from build123d import *

# Parameters (mm, degrees)
EXTRUDE_1_DEPTH = 10
SKETCH_2_R      = 10
EXTRUDE_2_DEPTH = 10


with BuildPart() as part:
    # 스케치1 → 보스-돌출1 (new body)
    with BuildSketch(Plane.XY):
        with BuildLine():
            Line((0, 20), (-82.363877474, 20))
            Line((-82.363877474, 20), (-82.363877474, -20))
            Line((-82.363877474, -20), (0, -20))
            ThreePointArc((0, -20), (20, 0), (0, 20))
        make_face()
    extrude(amount=EXTRUDE_1_DEPTH)

    # 스케치2 → 보스-돌출2 (add)
    with BuildSketch(Plane.XY.offset(10)):
        with Locations((0, -0.593223752)):
            Circle(SKETCH_2_R)
    extrude(amount=EXTRUDE_2_DEPTH)


solid = part.part
Build history of the part. All positions in model axes, mm. A direction names the side the tool comes from. Round coordinates to 2 decimals unless told otherwise and drop trailing zeros. Loops run counter-clockwise (first coordinate to the right, second up) from the corner with the lowest first, then second, coordinate; pieces in that order, holes last. Notation, with made-up numbers: (83.25, 29.25) -> (128.25, 29.25) arc R25 ccw to (128.25, 44.25) -> close; hole circle Ø2 at (-35.5, 55). An arc over 180 degrees is marked (long way). Use CSV: the item, a comma, the result in double quotes. Start each with the question number.
Q1. Saw through at A-A on x = 3.5. Give the cut face in (y, z), and give its area (3 significant figures).
Q2. Drill centre lines: L1, parallel to Z at x = -29.5, y = 13.5; L2, parallel to X at y = -0.5, z = 16; L3, parallel to X at y = 7, z = 7.5 (3 decimals). Where is each one in solid material? Low to high.
Q3. Saw through at D-D on x = -68.5. Give the cut face in (y, z).
Q4. Which spindle directions (+Z, -Z, +X, -X, +Y, -Y) get a long thin tool onto all of the face, cutting with end or side? Do faces 1 (the face through (-42, -20, 5)), 2 (the face through (-2.168, -10.355, 14.93)). Say none if no direction does.
Q5. Flat gauge pins, fed straight in: pin 1 Ø10 at (x, y) = (-53, 3.5) entering from +Z; pin 2 Ø1.5 at (y, z) = (10.5, 4) entering from +X; pin 3 Ø12 at (x, z) = (-15.5, 14.5) entering from +Y. Where does each tip first touch, or does it go through?
Q6. Saw through at C-C on z = 9. Give the cut face in (x, y), and give its area (3 significant figures).
Q7. Saw through at B-B on y = -2. Give the cut face in (x, z).
Solutions:
1,outline,"(-19.69, 0) -> (19.69, 0) -> (19.69, 10) -> (8.77, 10) -> (8.77, 20) -> (-9.96, 20) -> (-9.96, 10) -> (-19.69, 10) -> close"
1,area,"581 mm^2"
2,L1,"z = 0 to 10"
2,L2,"x = -10 to 10"
2,L3,"x = -82.364 to 18.735"
3,outline,"(-20, 0) -> (20, 0) -> (20, 10) -> (-20, 10) -> close"
4,face 1,"+Z, -Z, +X, -X, -Y"
4,face 2,"+Z"
5,pin 1,"stops at z = 10"
5,pin 2,"stops at x = 17.46"
5,pin 3,"stops at y = 20"
6,outline,"(-82.36, -20) -> (0, -20) arc R20 ccw to (0, 20) -> (-82.36, 20) -> close"
6,area,"3,920 mm^2"
7,outline,"(-82.36, 0) -> (19.9, 0) -> (19.9, 10) -> (9.9, 10) -> (9.9, 20) -> (-9.9, 20) -> (-9.9, 10) -> (-82.36, 10) -> close"
